from build123d import *

# Parameters (mm, degrees)
BOSS_EXTRUDE1_DEPTH = 10
SKETCH2_R           = 2
CUT_EXTRUDE1_DEPTH  = 20


with BuildPart() as part:
    # Sketch1 → Boss-Extrude1 (new body)
    with BuildSketch(Plane(origin=(0, 0, 0), x_dir=(1, 0, 0), z_dir=(0, 1, 0))):
        with BuildLine():
            Line((25, 0), (-25, 0))
            Line((-25, 0), (-25, 5))
            Line((-25, 5), (-15, 5))
            Line((-15, 5), (-15, 19))
            Line((-15, 19), (-6, 19))
            ThreePointArc((-6, 19), (0, 13), (6, 19))
            Line((6, 19), (15, 19))
            Line((15, 19), (15, 5))
            Line((15, 5), (25, 5))
            Line((25, 5), (25, 0))
        make_face()
    extrude(amount=BOSS_EXTRUDE1_DEPTH)

    # Sketch2 → Cut-Extrude1 (cut, through all)
    with BuildSketch(Plane.XY):
        with Locations((-20, 5)):
            Circle(SKETCH2_R)
        with Locations((-11, 5)):
            Circle(SKETCH2_R)
        with Locations((20, 5)):
            Circle(SKETCH2_R)
        with Locations((11, 5)):
            Circle(SKETCH2_R)
    extrude(amount=-CUT_EXTRUDE1_DEPTH, mode=Mode.SUBTRACT)


solid = part.part
Source: CAD feature listing. Evaluate the final solid. Frame: model axes, mm. A direction names the side the tool comes from. Round coordinates to 2 decimals unless told otherwise and drop trailing zeros. Loops run counter-clockwise (first coordinate to the right, second up) from the corner with the lowest first, then second, coordinate; pieces in that order, holes last. Notation, with made-up numbers: (-39.75, -33.5) - (-25.75, -33.5) arc R8 ccw to (-25.75, -21.5) - close; hole circle Ø1 at (29.25, 76.25). An arc over 180 degrees is marked (long way). Write item = value, one per line. Start each with the question number.
(1) Pull-direction query (Y, two-part tool) for faces 1 (the face through (0, 10, -8)), 2 (the face through (-15, 5, -12)), 3 (the face through (-22, 5, -2)); classes: +Y half, -Y half, draft (parallel to the pull), parting line (faces both ways), or undercut.
(2) Section query D-D, the plane z = -2.5. Output: boundary loops of the cut face in (x, y).
(3) Section query A-A, the plane x = 20. Output: boundary loops of the cut face in (y, z).
(4) Section query B-B, the plane y = 5. Output: boundary loops of the cut face in (x, z), plus the area to 3 significant figures.
(5) Section query C-C, the plane z = -8.25. Output: boundary loops of the cut face in (x, y), plus the area to 3 significant figures.
(6) Ray query, line 1 along Y through (x, z) = (-11, -13.25); line 2 along X through (y, z) = (5.5, -12.5); line 3 along X through (y, z) = (8, -6.75). Return the intervals inside material, ascending. Write a range as from..to.
(7) Set-up query: faces 4 (the face through (17.7, 4.9, -5)), 5 (the face through (-22.3, 4.9, -5)), 6 (the face through (0, 5, -13)). Return all of +Z, -Z, +X, -X, +Y, -Y with unobstructed straight access to the full face (end or side cutting, diameter ignored); none if empty.
(8) Pin query (flat end, axial travel): pin 1 (3 mm diameter, centred on y = 3.5, z = -14, fed in from -X); pin 2 (3 mm diameter, centred on x = 3.5, y = 7, fed in from -Z); pin 3 (5 mm diameter, centred on y = 4, z = -9, fed in from +X). Return the tip coordinate at first contact, or that it passes through.
Conclusion:
q1.face_1 = +Y half
q1.face_2 = draft
q1.face_3 = undercut
q2.outline = (-25, 0) - (25, 0) - (25, 10) - (-25, 10) - close; hole circle Ø4 at (-20, 5); hole circle Ø4 at (-11, 5); hole circle Ø4 at (11, 5); hole circle Ø4 at (20, 5)
q3.outline = (0, -5) - (3, -5) - (3, 0) - (0, 0) - close; (7, -5) - (10, -5) - (10, 0) - (7, 0) - close
q4.outline = (-25, -5) - (-22, -5) - (-22, 0) - (-25, 0) - close; (-18, -5) - (-15, -5) - (-15, -19) - (-13, -19) - (-13, 0) - (-18, 0) - close; (-9, -19) - (-6, -19) arc R6 cw to (6, -19) - (9, -19) - (9, 0) - (-9, 0) - close; (13, -19) - (15, -19) - (15, -5) - (18, -5) - (18, 0) - (13, 0) - close; (22, -5) - (25, -5) - (25, 0) - (22, 0) - close
q4.area = 421 mm2
q5.outline = (-15, 0) - (15, 0) - (15, 10) - (-15, 10) - close; hole circle Ø4 at (-11, 5); hole circle Ø4 at (11, 5)
q5.area = 275 mm2
q6.line_1 = 0..3, 7..10
q6.line_2 = -15..-12.94, -9.06..9.06, 12.94..15
q6.line_3 = -15..15
q7.face_4 = -Z, +X, +Y, -Y
q7.face_5 = -Z, -X, +Y, -Y
q7.face_6 = -Z, +Y, -Y
q8.pin_1 = -15
q8.pin_2 = -15.68
q8.pin_3 = 15
